from build123d import *

# Parameters (mm, degrees)
SKETCH1_W               = 52
SKETCH1_H               = 58
SKETCH1_W_2             = 32
SKETCH1_H_2             = 32
BOSS_EXTRUDE1_DEPTH     = 3
SKETCH2_W               = 52
SKETCH2_H               = 58
SKETCH2_W_2             = 42
SKETCH2_H_2             = 42
BOSS_EXTRUDE2_DEPTH     = 4
SKETCH3_W               = 8
SKETCH3_H               = 8
BOSS_EXTRUDE3_DEPTH     = 23.5
SKETCH4_R               = 2.25
CUT_EXTRUDE1_DEPTH      = 50.469687689
SKETCH5_W               = 5.3
SKETCH5_H               = 5.3
CUT_EXTRUDE2_DEPTH      = 15
MIRROR2_COPY_1_SKETCH_W = 8
MIRROR2_COPY_1_SKETCH_H = 8
MIRROR2_COPY_1_DEPTH    = 23.5
MIRROR2_COPY_2_SKETCH_R = 2.25
MIRROR2_COPY_2_DEPTH    = 50.469687689
MIRROR2_COPY_3_SKETCH_W = 5.3
MIRROR2_COPY_3_SKETCH_H = 5.3
MIRROR2_COPY_3_DEPTH    = 15
SKETCH6_W               = 2
SKETCH6_H               = 0.75
SKETCH6_W_2             = 0.75
SKETCH6_H_2             = 2
BOSS_EXTRUDE4_DEPTH     = 4
SKETCH7_W               = 4.25
SKETCH7_H               = 2
SKETCH7_W_2             = 2
SKETCH7_H_2             = 4.25
BOSS_EXTRUDE5_DEPTH     = 2
CUT_EXTRUDE3_REACH      = 51.47
SKETCH8_W               = 42
SKETCH8_H               = 2
BOSS_EXTRUDE6_DEPTH     = 20
SKETCH10_W              = 8
SKETCH10_H              = 10
SKETCH10_R              = 2.25
BOSS_EXTRUDE7_DEPTH     = 8
SKETCH11_W              = 10
SKETCH11_H              = 8
CUT_EXTRUDE4_DEPTH      = 2
BOSS_EXTRUDE8_DEPTH     = 2.5
FILLET1_R               = 1


with BuildPart() as part:
    # Sketch1 → Boss-Extrude1 (new body)
    with BuildSketch(Plane(origin=(0, 0, 0), x_dir=(0, 0, -1), z_dir=(1, 0, 0))):
        Rectangle(SKETCH1_W, SKETCH1_H)
        Rectangle(SKETCH1_W_2, SKETCH1_H_2, mode=Mode.SUBTRACT)
    extrude(amount=-BOSS_EXTRUDE1_DEPTH)

    # Sketch2 → Boss-Extrude2 (add)
    with BuildSketch(Plane.ZY.offset(3)):
        Rectangle(SKETCH2_W, SKETCH2_H)
        Rectangle(SKETCH2_W_2, SKETCH2_H_2, mode=Mode.SUBTRACT)
    extrude(amount=BOSS_EXTRUDE2_DEPTH)

    # Sketch3 → Boss-Extrude3 (add)
    with BuildSketch(Plane.ZY.offset(7)):
        with Locations((-22, 25)):
            Rectangle(SKETCH3_W, SKETCH3_H)
    boss_extrude3 = extrude(amount=BOSS_EXTRUDE3_DEPTH)

    # Sketch4 → Cut-Extrude1 (cut, through all)
    with BuildSketch(Plane(origin=(0, 0, 0), x_dir=(0, 0, -1), z_dir=(1, 0, 0))):
        with Locations((22, 25)):
            Circle(SKETCH4_R)
    cut_extrude1 = extrude(amount=-CUT_EXTRUDE1_DEPTH, mode=Mode.SUBTRACT)

    # Sketch5 → Cut-Extrude2 (cut)
    with BuildSketch(Plane.ZY.offset(30.5)):
        with Locations((-23.35, 26.35)):
            Rectangle(SKETCH5_W, SKETCH5_H)
    cut_extrude2 = extrude(amount=-CUT_EXTRUDE2_DEPTH, mode=Mode.SUBTRACT)

    # Mirror1: Boss-Extrude3, Cut-Extrude1, Cut-Extrude2 across plane
    add(boss_extrude3.mirror(Plane.ZX))
    add(cut_extrude1.mirror(Plane.ZX), mode=Mode.SUBTRACT)
    add(cut_extrude2.mirror(Plane.ZX), mode=Mode.SUBTRACT)

    # Mirror2: Boss-Extrude3, Cut-Extrude1, Cut-Extrude2 across plane
    add(boss_extrude3.mirror(Plane.XY))
    add(cut_extrude1.mirror(Plane.XY), mode=Mode.SUBTRACT)
    add(cut_extrude2.mirror(Plane.XY), mode=Mode.SUBTRACT)

    # Mirror2 copy 1 sketch → Mirror2 copy 1 (add)
    with BuildSketch(Plane(origin=(-7, 0, 0), x_dir=(0, 0, -1), z_dir=(-1, 0, 0))):
        with Locations((-22, 25)):
            Rectangle(MIRROR2_COPY_1_SKETCH_W, MIRROR2_COPY_1_SKETCH_H)
    extrude(amount=MIRROR2_COPY_1_DEPTH)

    # Mirror2 copy 2 sketch → Mirror2 copy 2 (cut, through all)
    with BuildSketch(Plane(origin=(0, 0, 0), x_dir=(0, 0, 1), z_dir=(1, 0, 0))):
        with Locations((22, 25)):
            Circle(MIRROR2_COPY_2_SKETCH_R)
    extrude(amount=-MIRROR2_COPY_2_DEPTH, mode=Mode.SUBTRACT)

    # Mirror2 copy 3 sketch → Mirror2 copy 3 (cut)
    with BuildSketch(Plane(origin=(-30.5, 0, 0), x_dir=(0, 0, -1), z_dir=(-1, 0, 0))):
        with Locations((-23.35, 26.35)):
            Rectangle(MIRROR2_COPY_3_SKETCH_W, MIRROR2_COPY_3_SKETCH_H)
    extrude(amount=-MIRROR2_COPY_3_DEPTH, mode=Mode.SUBTRACT)

    # Sketch6 → Boss-Extrude4 (add)
    with BuildSketch(Plane.ZY.offset(3)):
        with Locations((-13.2, 20.625)):
            Rectangle(SKETCH6_W, SKETCH6_H)
        with Locations((-4.4, 20.625)):
            Rectangle(SKETCH6_W, SKETCH6_H)
        with Locations((4.4, 20.625)):
            Rectangle(SKETCH6_W, SKETCH6_H)
        with Locations((13.2, 20.625)):
            Rectangle(SKETCH6_W, SKETCH6_H)
        with Locations((20.625, 13.2)):
            Rectangle(SKETCH6_W_2, SKETCH6_H_2)
        with Locations((20.625, 4.4)):
            Rectangle(SKETCH6_W_2, SKETCH6_H_2)
        with Locations((-20.625, 13.2)):
            Rectangle(SKETCH6_W_2, SKETCH6_H_2)
        with Locations((-20.625, 4.4)):
            Rectangle(SKETCH6_W_2, SKETCH6_H_2)
    boss_extrude4 = extrude(amount=BOSS_EXTRUDE4_DEPTH)

    # Sketch7 → Boss-Extrude5 (add)
    with BuildSketch(Plane.ZY.offset(3)):
        with Locations((-18.125, 4.4)):
            Rectangle(SKETCH7_W, SKETCH7_H)
        with Locations((-18.125, 13.2)):
            Rectangle(SKETCH7_W, SKETCH7_H)
        with Locations((-13.2, 18.125)):
            Rectangle(SKETCH7_W_2, SKETCH7_H_2)
        with Locations((-4.4, 18.125)):
            Rectangle(SKETCH7_W_2, SKETCH7_H_2)
        with Locations((4.4, 18.125)):
            Rectangle(SKETCH7_W_2, SKETCH7_H_2)
        with Locations((13.2, 18.125)):
            Rectangle(SKETCH7_W_2, SKETCH7_H_2)
        with Locations((18.125, 13.2)):
            Rectangle(SKETCH7_W, SKETCH7_H)
        with Locations((18.125, 4.4)):
            Rectangle(SKETCH7_W, SKETCH7_H)
    boss_extrude5 = extrude(amount=BOSS_EXTRUDE5_DEPTH)

    # Mirror3: Boss-Extrude4, Boss-Extrude5 across plane
    add(boss_extrude4.mirror(Plane.ZX))
    add(boss_extrude5.mirror(Plane.ZX))

    # Cut-Extrude3: up to this face of the body (flat: up to its plane)
    cut_extrude3_end = Plane(part.part.faces().sort_by_distance((-5, 18.125, -13.2))[0])
    # Sketch8 → Cut-Extrude3 (cut, up to the picked face)
    with BuildSketch(Plane.ZY.offset(30.5), mode=Mode.PRIVATE) as cut_extrude3_sk1:
        with Locations((0, 21.25)):
            Rectangle(SKETCH8_W, SKETCH8_H)
    cut_extrude3_tool1 = split(extrude(cut_extrude3_sk1.sketch, amount=-CUT_EXTRUDE3_REACH, mode=Mode.PRIVATE), bisect_by=cut_extrude3_end, keep=Keep.BOTH, mode=Mode.PRIVATE)
    add(cut_extrude3_tool1.solids().sort_by(Axis((-30.5, 21.25, 0), (1, 0, 0)))[0], mode=Mode.SUBTRACT)

    # Sketch9 → Boss-Extrude6 (add)
    with BuildSketch(Plane.ZY.offset(3)):
        Polygon((-22, -21), (-22, -19), (-20.25, -19), (-20.25, -20.25), (-19, -20.25), (-19, -21), align=None)
    boss_extrude6 = extrude(amount=BOSS_EXTRUDE6_DEPTH)

    # Mirror4: Boss-Extrude6 across plane
    add(boss_extrude6.mirror(Plane.XY))

    # Sketch10 → Boss-Extrude7 (add)
    with BuildSketch(Plane.XZ.offset(29)):
        with Locations((-4, 31)):
            Rectangle(SKETCH10_W, SKETCH10_H)
        with Locations(Location((-4, 32, 0), (0, 0, 270))):
            Circle(SKETCH10_R, mode=Mode.SUBTRACT)
    boss_extrude7 = extrude(amount=-BOSS_EXTRUDE7_DEPTH)

    # Mirror5: Boss-Extrude7 across plane
    add(boss_extrude7.mirror(Plane.XY))

    # Sketch11 → Cut-Extrude4 (cut)
    with BuildSketch(Plane.ZY.offset(7)):
        with Locations((-6, 26.25)):
            Rectangle(SKETCH11_W, SKETCH11_H)
    extrude(amount=-CUT_EXTRUDE4_DEPTH, mode=Mode.SUBTRACT)

    # Sketch12 → Boss-Extrude8 (add)
    with BuildSketch(Plane.XZ.offset(29)):
        Polygon((-15.5, 20.7), (-30.5, 20.7), (-30.5, 18), (-7, 18), (-7, -18), (-30.5, -18), (-30.5, -20.7), (-15.5, -20.7), (-15.5, -26), (-8, -26), (-8, -36), (0, -36), (0, 36), (-8, 36), (-8, 26), (-15.5, 26), align=None)
    extrude(amount=BOSS_EXTRUDE8_DEPTH)

    # Fillet1
    fillet1_edges = [part.edges().sort_by_distance(p)[0] for p in [
        (0, 29, 0),
        (0, 4, 26),
        (0, -21, 31),
        (0, -26.25, 36),
        (0, 4, -26),
        (0, -26.25, -36),
        (0, -21, -31),
        (0, -31.5, 0),
    ]]
    fillet(fillet1_edges, radius=FILLET1_R)


solid = part.part
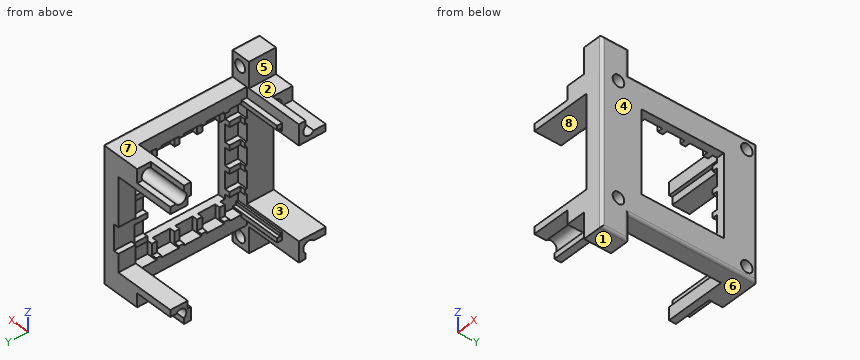
Read the model definition and answer for the solid it produces. Units are mm, in the model's axes. Face numbers are marked on the shaded views. A direction names the side the tool comes from. Give positions to 0.01 mm unless a question says otherwise; leave off trailing zeros. Write each loop counter-clockwise with the first axis right and the second up, starting at its lowest first coordinate (ties: lowest second). Pieces come first, ordered by that corner, then holes. Notation, with made-up numbers: (13.5, 39) -> (17.5, 39) arc R22 cw to (17.5, 48) -> close; hole circle Ø4 at (29.5, 29.25). An arc over 180 degrees is marked (long way). Answer as a JSON object with one key per item and string values. Group by question number.
1) Find section A-A (y = -25). Write down the section's boundary in (x, z), and give its area (3 significant figures).
2) Find section C-C (y = -0.5). Write down the section's boundary in (x, z).
3) The mould has two halves that part along Z. Classify the marked faces 1, 2, 3 and 4: +Z half, -Z half, draft (parallel to the pull), parting line (faces both ways), or undercut.
4) Find section B-B (x = -24). Count the separate pieces of the cut face and the enclosed holes in it, and give its area (3 significant figures).
5) A tool of negligible diameter and unlimited length cuts with its end or side. For the marked faces 5, 6, 7 and 8, from which of +Z, -Z, +X, -X, +Y, -Y can it reach the whole face along a straight path? Write none if from no direction.
6) Each of these flat-tipped pins is pushed along its axis until it touches: P1, Ø10, axis at x = -16.5, y = -20, coming from the +Z side; P2, Ø2, axis at x = -5.5, y = -17.5, coming from the -Z side; P3, Ø2, axis at y = -18.5, z = 19, coming from the -X side. Where does it stop, or does it pass through?
7) Consider L1, parallel to Z at x = -8.5, y = -25; L2, parallel to Z at x = -23, y = -25; L3, parallel to X at y = -23, z = 32. Determine where each line is inside the solid, lowest interval first. Write a range as from..to.
8) Find section D-D (z = -17). Write down the section's boundary in (x, y), and give its area (3 significant figures).
Values follow:
{
 "1": {"outline": "(-30.5, -19.75) -> (0, -19.75) -> (0, 19.75) -> (-30.5, 19.75) -> (-30.5, 18) -> (-7, 18) -> (-7, -18) -> (-30.5, -18) -> close; (-15.5, -26) -> (-8, -26) -> (-8, -36) -> (-1, -36) arc R1 ccw to (0, -35) -> (0, -24.25) -> (-15.5, -24.25) -> close; (-15.5, 24.25) -> (0, 24.25) -> (0, 35) arc R1 ccw to (-1, 36) -> (-8, 36) -> (-8, 26) -> (-15.5, 26) -> close; hole circle Ø4.5 at (-4, -32); hole circle Ø4.5 at (-4, 32)", "area": "541 mm2"},
 "2": {"outline": "(-7, -26) -> (-1, -26) arc R1 ccw to (0, -25) -> (0, -16) -> (-3, -16) -> (-3, -21) -> (-7, -21) -> close; (-7, 21) -> (-3, 21) -> (-3, 16) -> (0, 16) -> (0, 25) arc R1 ccw to (-1, 26) -> (-7, 26) -> close"},
 "3": {"face 1": "-Z half", "face 2": "+Z half", "face 3": "undercut", "face 4": "draft"},
 "4": {"separate pieces": "4", "enclosed holes": "0", "area": "131 mm2"},
 "5": {"face 5": "+Z, -X, +Y, -Y", "face 6": "-Z, +X, -X, +Y", "face 7": "+Z, +X, -X, +Y", "face 8": "-X, +Y, -Y"},
 "6": {"P1": "stops at z = 26", "P2": "stops at z = -26", "P3": "stops at x = -3"},
 "7": {"L1": "z = -26..-24.25, -19.75..-18, 18..19.75, 24.25..26", "L2": "z = -19.75..-18, 18..19.75", "L3": "x = -8..-6.25, -1.75..0"},
 "8": {"outline": "(-7, -31.5) -> (-1, -31.5) arc R1 ccw to (0, -30.5) -> (0, 28) arc R1 ccw to (-1, 29) -> (-7, 29) -> (-7, 22.25) -> (-5, 22.25) -> (-5, 21) -> (-3, 21) -> (-3, 14.2) -> (-5, 14.2) -> (-5, 12.2) -> (-3, 12.2) -> (-3, 5.4) -> (-5, 5.4) -> (-5, 3.4) -> (-3, 3.4) -> (-3, -3.4) -> (-5, -3.4) -> (-5, -5.4) -> (-3, -5.4) -> (-3, -12.2) -> (-5, -12.2) -> (-5, -14.2) -> (-3, -14.2) -> (-3, -21) -> (-7, -21) -> close", "area": "269 mm2"}
}
